from build123d import *

# Parameters (mm, degrees)
F0_R      = 8
F1_DEPTH  = 4.8
F2_R      = 6
F3_DEPTH  = 4.6
F4_R      = 8
F5_DEPTH  = 30.6
F6_SIZE   = 2
F7_R      = 3
F8_DEPTH  = 2
F9_W      = 21.1684573442
F9_H      = 14.4873037934
F10_DEPTH = 10
F11_R     = 5
F12_DEPTH = 5
F12_TAPER = 45
F13_R     = 6
F14_DEPTH = 10


with BuildPart() as f1:
    # F0 (on Top) → F1 (new body)
    with BuildSketch(Plane.XY):
        Circle(F0_R)
    extrude(amount=F1_DEPTH)

    # F2 (on face) → F3 (join)
    with BuildSketch(Plane.XY.offset(4.8)):
        Circle(F2_R)
    extrude(amount=F3_DEPTH)

    # F4 (on face) → F5 (join)
    with BuildSketch(Plane.XY.offset(9.4)):
        Circle(F4_R)
    extrude(amount=F5_DEPTH)

    # F6
    f6_edges = [f1.edges().sort_by_distance(p)[0] for p in [
        (-8, 0, 40),
    ]]
    chamfer(f6_edges, length=F6_SIZE)

    # F7 (on face) → F8 (join)
    with BuildSketch(Plane.XY.offset(40)):
        Circle(F7_R)
    extrude(amount=F8_DEPTH)

    # F9 (on face) → F10 (join)
    with BuildSketch(Plane.XY.offset(42)):
        with Locations((0.0396473333, -1.0394603014)):
            Rectangle(F9_W, F9_H)
    extrude(amount=F10_DEPTH)

    # F11 (on face) → F12 (join)
    with BuildSketch(Plane.XY.offset(52)):
        Circle(F11_R)
    extrude(amount=F12_DEPTH, taper=F12_TAPER)

    # F13 (on face) → F14 (join)
    with BuildSketch(Plane(origin=(0, 0, 0), x_dir=(1, 0, 0), z_dir=(0, 0, -1))):
        Circle(F13_R)
    extrude(amount=F14_DEPTH)


solid = f1.part
The listing builds one solid part. Answer for the finished solid, in the listing's coordinates (mm). A direction names the side the tool comes from. Round coordinates to 2 decimals unless told otherwise and drop trailing zeros. Loops run counter-clockwise (first coordinate to the right, second up) from the corner with the lowest first, then second, coordinate; pieces in that order, holes last. Notation, with made-up numbers: M 50,88.25 L 71,88.25 A31 ccw 71,118.25 Z; hole C 59,55 d1. An arc over 180 degrees is marked long. Write each question's results on one line, items separated by ' | '. Start each with the question number.
1) Find section B-B on x = -7. Count the separate pieces of the cut face and the enclosed holes in it, plus the area to 3 significant figures.
2) Find section A-A on z = 22. Write down the section's boundary in (x, y).
3) Which of the six approach directions +Z, -Z, +X, -X, +Y, -Y give full straight-line access (tool end or side, diameter ignored) to faces 1 (the flat face through (0, 6.204, 47)), 2 (the cylindrical face through (-1.73, -7.81, 2.37)), 3 (the cylindrical face through (-6, 0, 7))?
4) Determine the mould class of faces 4 (the cylindrical face through (-6, 0, -5)), 5 (the conical face through (0, 1, 56)), 6 (the flat face through (-2, 6, 4.8)) for opening direction Z: pulls with the +Z half, pulls with the -Z half, needs draft (parallel to the pull), parting line crosses it, or undercut.
5) Each of these flat-tipped pins is pushed along its axis until it touches: pin 1 (11 mm diameter, centred on x = -2, z = 47, fed in from +Y); pin 2 (7 mm diameter, centred on x = -1.5, y = -4, fed in from +Z); pin 3 (5 mm diameter, centred on x = -2.5, y = 4, fed in from +Z); pin 4 (4 mm diameter, centred on x = 0.5, z = 35, fed in from +Y). Where does it stop, or does it pass through?
6) Straight lines are drawn through the part: probe 1 along Z at (x, y) = (3, 4.5); probe 2 along Z at (x, y) = (7, 0); probe 3 along Z at (x, y) = (-6, -5.25). For each, find the intervals that lie inside material, in ascending order.
Final values:
1) separate pieces: 3 | enclosed holes: 0 | area: 409 mm²
2) outline: C 0,0 d16
3) face 1: +Z, +X, -X, +Y | face 2: -Z | face 3: none
4) face 4: needs draft | face 5: pulls with the +Z half | face 6: undercut
5) pin 1: y = 6.2 | pin 2: z = 56.23 | pin 3: z = 54.78 | pin 4: y = 8
6) probe 1: -10 to 40, 42 to 52 | probe 2: 0 to 4.8, 9.4 to 39, 42 to 52 | probe 3: 0 to 4.8, 9.4 to 38.03, 42 to 52
